Design review of the part shown in the three views and the two pictorial views. Dimensions are in mm from the part's minimum x, y and z. Round coordinates to 2 decimals unless told otherwise and drop trailing zeros. Loops run counter-clockwise (first coordinate to the right, second up) from the corner with the lowest first, then second, coordinate; pieces in that order, holes last. Notation, with made-up numbers: (38.25, -29.75) -> (65.25, -29.75) arc R31 cw to (65.25, 0.25) -> close; hole circle Ø10 at (80.5, 62). An arc over 180 degrees is marked (long way). Write each question's results on one line, items separated by ' | '. Start each with the question number.
Item 1: For L1, parallel to Y at x = 333, z = 1.9; L2, parallel to X at y = 9.5, z = 2.75; L3, parallel to X at y = 3.5, z = 4, list the stretches that pass through material, from the lowest coordinate up. Write a range as from..to.
Item 2: We need section A-A (z = 2.25). Give the number of separate pieces and of enclosed holes in the cut face, and give its area (3 significant figures).
Item 3: We need section B-B (x = 205.5). Give the boundary of the cut face in (y, z).
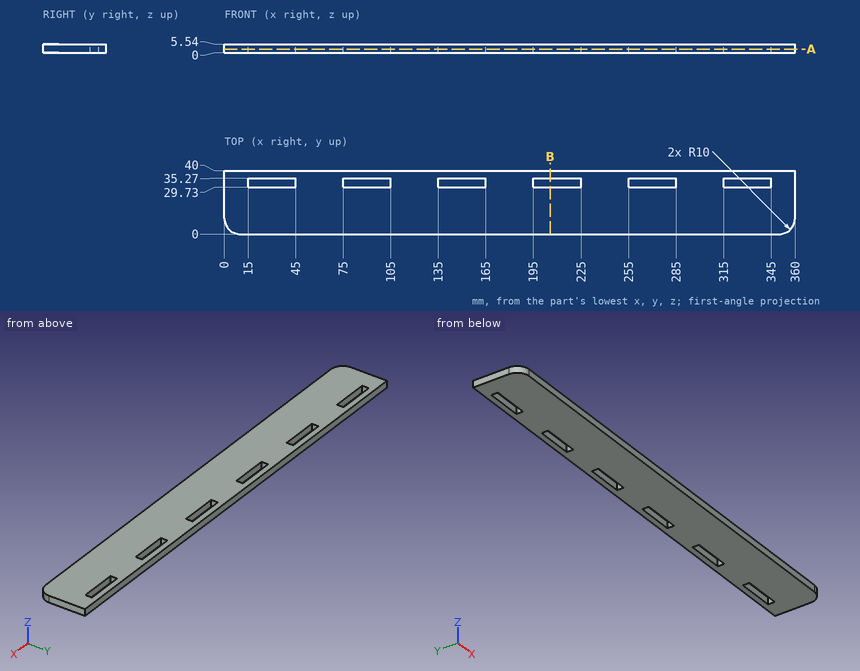
Here are the results:
1) L1: y = 0..29.73, 35.27..40 | L2: x = 0.01..359.99 | L3: x = 2.4..357.6
2) separate pieces: 1 | enclosed holes: 6 | area: 13,400 mm2
3) outline: (0, 0) -> (29.73, 0) -> (29.73, 5.54) -> (0, 5.54) -> close; (35.27, 0) -> (40, 0) -> (40, 5.54) -> (35.27, 5.54) -> close
